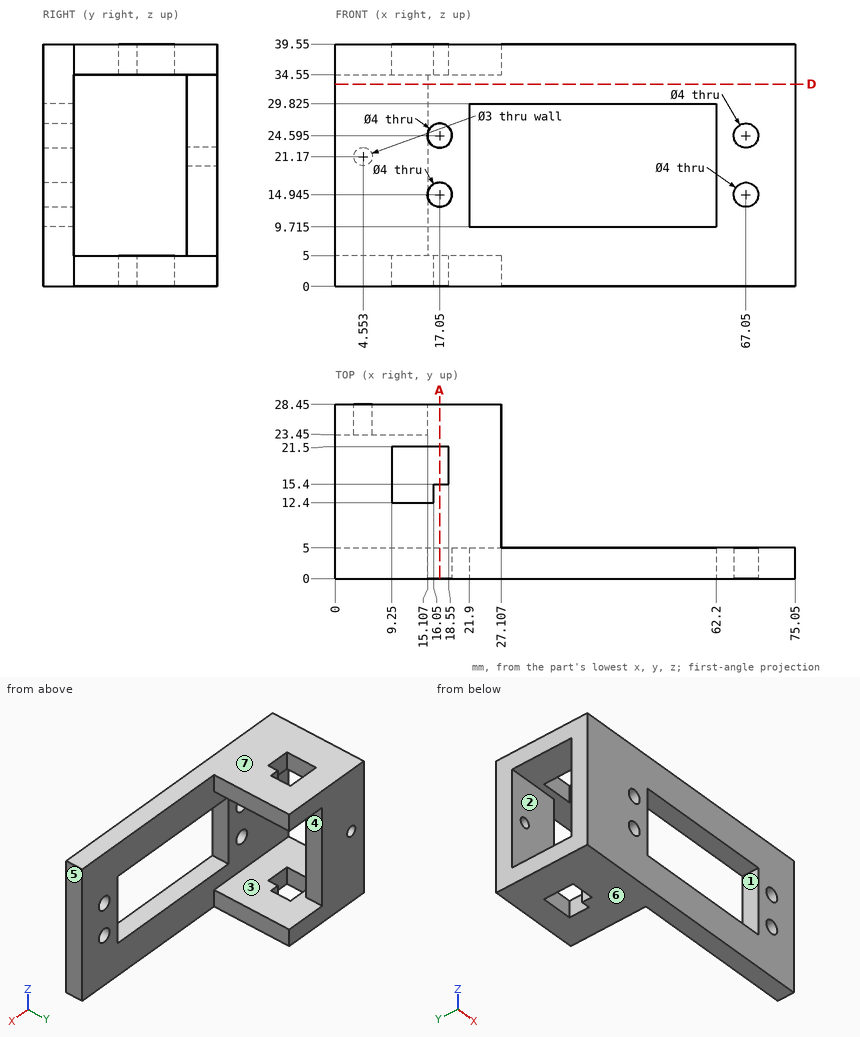
Answer from the drawing. Dimensions are ordinates in mm from the lowest x, y and z of the part. A direction names the side the tool comes from. Round coordinates to 2 decimals unless told otherwise and drop trailing zeros. Order: outer loops, then holes, each group sorted by start corner. A loop starts at its lowest first (then second) coordinate and runs counter-clockwise, first axis right, second up. Notation, with made-up numbers: (42.5, 14.25) - (77.5, 14.25) arc R30 ccw to (77.5, 44.25) - close; hole circle Ø1 at (-22, 9). An arc over 180 degrees is marked (long way). Put each result on its own line as item: value. Start each with the question number.
(1) Find section D-D (z = 33). Give the vertices of the cut face in (x, y).
(2) Determine the mould class of the marked faces 4, 5, 6 and 7 for opening direction Z: released by +Z, released by -Z, zero draft, split by the parting line, or undercut.
(3) Straight lines are drawn through the part: probe 1 along X at (y, z) = (3, 19.5); probe 2 along Z at (x, y) = (4, 17.5); probe 3 along X at (y, z) = (25.6, 21.17). For each, find the intervals that lie inside material, in ascending order. Write a range as from..to.
(4) For the marked faces 1, 2 and 3, determine the directions among +Z, -Z, +X, -X, +Y, -Y from which every point of the face is accessible in a straight line to the end or side of a thin tool.
(5) Given P1, Ø1.5, axis at y = 16, z = 2, coming from the +X side; P2, Ø20, axis at x = 40.5, z = 17, coming from the +Y side, each flat-ended and moving along its own axis, determine where each tip first touches the part or whether it passes through.
(6) Find section A-A (x = 17.05). State how many separate pieces and enclosed holes the cut face has, plus the area to 3 significant figures.
Reply:
1. outline: (0, 0) - (75.05, 0) - (75.05, 5) - (0, 5) - close; (0, 23.45) - (15.11, 23.45) - (15.11, 28.45) - (0, 28.45) - close
2. face 4: undercut
2. face 5: zero draft
2. face 6: released by -Z
2. face 7: released by +Z
3. probe 1: 0..21.9, 62.2..75.05
3. probe 2: 0..5, 34.55..39.55
3. probe 3: 0..3.05, 6.05..15.11
4. face 1: +Y, -Y
4. face 2: +X, -X
4. face 3: +X
5. P1: x = 27.11
5. P2: y = 5
6. separate pieces: 5
6. enclosed holes: 0
6. area: 331 mm^2
